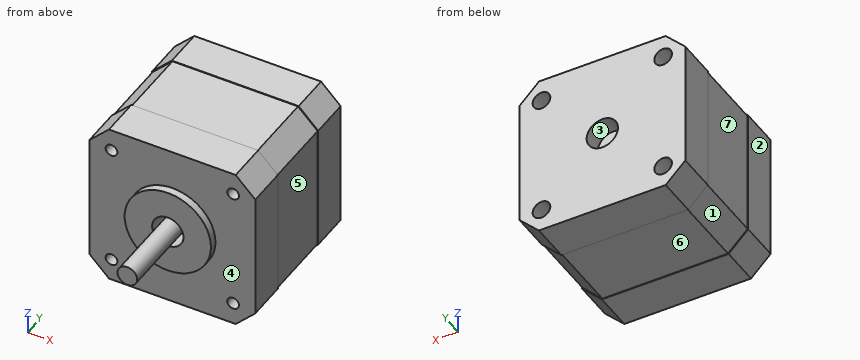
Solid Edge part; units mm, degrees
sketch "Sketch1" plane through (0, 0, 0) normal (0, -1, 0) x (1, 0, 0)
  line L0 (-5.4714, -0.2002) -> (36.8286, -0.2002)
  line L1 (36.8286, -0.2002) -> (36.8286, 42.0998)
  line L2 (36.8286, 42.0998) -> (-5.4714, 42.0998)
  line L3 (-5.4714, 42.0998) -> (-5.4714, -0.2002)
extrude "Protrusion1" add sketch "Sketch1" against normal blind 10
sketch "Sketch2" plane through (15.6786, 0, 20.9498) normal (0, -1, 0) x (1, 0, 0)
  circle A0 centre (0, 0) radius 11
extrude "ProtrusiónExtruida_2" add sketch "Sketch2" along normal blind 2
chamfer "Chaflán_2" distance 5 angle 45 4 edges at (36.8286, 5, 42.0998) (36.8286, 5, -0.2002) (-5.4714, 5, -0.2002) (-5.4714, 5, 42.0998)
sketch "Sketch3" plane through (15.6786, -2, 20.9498) normal (0, -1, 0) x (1, 0, 0)
  circle A0 centre (0, 0) radius 4
  circle A1 centre (15.5, 15.5) radius 1.5
  circle A2 centre (-15.5, 15.5) radius 1.5
  circle A3 centre (-15.5, -15.5) radius 1.5
  circle A4 centre (15.5, -15.5) radius 1.5
extrude "VaciadoExtruido_2" cut sketch "Sketch3" against normal blind 7
sketch "Sketch4" plane through (15.6786, 5, 20.9498) normal (0, -1, 0) x (1, 0, 0)
  circle A0 centre (0, 0) radius 2.5
extrude "ProtrusiónExtruida_3" add sketch "Sketch4" along normal blind 25
sketch "Sketch5" plane through (15.6786, 10, 20.9498) normal (0, 1, 0) x (0, 0, -1)
  line L0 (-21, -21) -> (21, -21)
  line L1 (21, -21) -> (21, 21)
  line L2 (21, 21) -> (-21, 21)
  line L3 (-21, 21) -> (-21, -21)
extrude "ProtrusiónExtruida_4" add sketch "Sketch5" along normal blind 18
chamfer "Chaflán_9" distance 5 angle 45 4 edges at (-5.3214, 19, 41.9498) (36.6786, 19, 41.9498) (36.6786, 19, -0.0502) (-5.3214, 19, -0.0502)
sketch "Sketch6" plane through (15.6786, 28, 20.9498) normal (0, 1, 0) x (0, 0, -1)
  line L0 (21.15, -21.15) -> (-21.15, -21.15)
  line L1 (-21.15, -21.15) -> (-21.15, 21.15)
  line L2 (-21.15, 21.15) -> (21.15, 21.15)
  line L3 (21.15, 21.15) -> (21.15, -21.15)
extrude "ProtrusiónExtruida_5" add sketch "Sketch6" along normal blind 10
chamfer "Chaflán_10" distance 5 angle 45 4 edges at (36.8286, 33, 42.0998) (-5.4714, 33, 42.0998) (-5.4714, 33, -0.2002) (36.8286, 33, -0.2002)
sketch "Sketch7" plane through (15.6786, 38, 20.9498) normal (0, 1, 0) x (-1, 0, 0)
  circle A0 centre (0, 0) radius 4
  circle A1 centre (-15.5, 15.5) radius 2.25
  circle A2 centre (15.5, 15.5) radius 2.25
  circle A3 centre (15.5, -15.5) radius 2.25
  circle A4 centre (-15.5, -15.5) radius 2.25
extrude "VaciadoExtruido_3" cut sketch "Sketch7" against normal blind 5
Design review of the part built by this model. Coordinates are the model's own, in mm. Face numbers are marked on the shaded views. A direction names the side the tool comes from. Coordinates: 2 decimals unless noted, no trailing zeros. Loops run counter-clockwise (first coordinate to the right, second up) from the corner with the lowest first, then second, coordinate; pieces in that order, holes last. Notation, with made-up numbers: M 7.25,-37.5 L 65.25,-37.5 A19 cw 65.25,-18.5 Z; hole C -17,34.25 d7. An arc over 180 degrees is marked long. Use one line per item in the form item = value.
(1) Consider section B-B (x = 4). Write out the cut boundary in (y, z).
Return value:
outline = M 0,-0.2 L 10,-0.2 L 10,-0.05 L 28,-0.05 L 28,-0.2 L 38,-0.2 L 38,42.1 L 28,42.1 L 28,41.95 L 10,41.95 L 10,42.1 L 0,42.1 Z
(2) Clearance check with flat-ended pins moving along their axes: P1, Ø1.3, axis at x = 0, z = 4.5, coming from the +Y side; P2, Ø4, axis at x = 0.18, z = 5.45, coming from the -Y side; P3, Ø2.5, axis at x = 31.18, z = 36.45, coming from the -Y side. State where each tip first meets the part, or that it passes through.
Return value:
P1 = 33
P2 = 0
P3 = 5
(3) For the marked faces 4, 5, 6 and 7, list the 3-axis set-ups (+Z, -Z, +X, -X, +Y, -Y) from which the entire face can be reached by the end or side of a thin tool; tool diameter is ignored.
Return value:
face_4 = -Y
face_5 = +Z, -Z, +X
face_6 = -Z, +X, -X
face_7 = +Z, -Z, -X
(4) Consider section A-A (y = 26). Write out the cut boundary in (x, z).
Return value:
outline = M -5.32,4.95 L -0.32,-0.05 L 31.68,-0.05 L 36.68,4.95 L 36.68,36.95 L 31.68,41.95 L -0.32,41.95 L -5.32,36.95 Z
(5) For line 1 along Z through (x, y) = (17, 2); line 2 along Y through (x, z) = (32, 32); line 3 along Z through (x, y) = (20, 21), list the stretches that pass through material, from the lowest coordinate up. Write a range as from..to.
Return value:
line_1 = -0.2..17.17, 18.83..23.07, 24.73..42.1
line_2 = 0..38
line_3 = -0.05..41.95
(6) Consider section D-D (z = 28.5). Write out the cut boundary in (x, y).
Return value:
outline = M -5.47,0 L 7.68,0 L 7.68,-2 L 23.68,-2 L 23.68,0 L 36.83,0 L 36.83,10 L 36.68,10 L 36.68,28 L 36.83,28 L 36.83,38 L -5.47,38 L -5.47,28 L -5.32,28 L -5.32,10 L -5.47,10 Z
(7) Draft analysis for pull direction Z (two halves, no side actions). For the marked faces 1, 2 and 3, state which applies: pulls with the +Z half, pulls with the -Z half, needs draft (parallel to the pull), parting line crosses it, or undercut.
Return value:
face_1 = pulls with the -Z half
face_2 = needs draft
face_3 = undercut
(8) Consider section C-C (y = -1). Write out the cut boundary in (x, z).
Return value:
outline = C 15.68,20.95 d22; C 15.68,20.95 d5; hole C 15.68,20.95 d8
